CAD build for the part. Positions are in the model's coordinates, mm. A direction names the side the tool comes from. Give positions to 0.01 mm unless a question says otherwise; leave off trailing zeros. Write each loop counter-clockwise with the first axis right and the second up, starting at its lowest first coordinate (ties: lowest second). Pieces come first, ordered by that corner, then holes. Notation, with made-up numbers: (44.5, 68) - (78.5, 68) arc R17 ccw to (78.5, 99) - close; hole circle Ø1 at (1.5, -34.5). An arc over 180 degrees is marked (long way). Put each result on its own line as item: value. Start each with the question number.
1. Cut at C-C on y = 10.5. List the corners of the cut face in (x, z), and give its area (3 significant figures).
2. Cut at A-A on x = -8. List the corners of the cut face in (y, z).
3. Cut at B-B on z = -89.5. List the corners of the cut face in (x, y).
4. Wall check: line 1 (Z direction, x = 11, y = 9.25); line 2 (Z direction, x = 15, y = 2.5); line 3 (X direction, y = 0.25, z = -55.5). Give the ranges that are in metal, low to high.
5. Drop flat-ended pins along their axis: pin 1 (3 mm diameter, centred on y = 4.5, z = -20.5, fed in from -X); pin 2 (1 mm diameter, centred on y = -9.5, z = -2, fed in from -X); pin 3 (0.6 mm diameter, centred on x = 3, z = 111.5, fed in from -Y). Give the stop position or say it passes through.
6. Tool access for faces 1 (the flat face through (0, 9, 110.5)), 2 (the cylindrical face through (17, 0, 111)), 3 (the cylindrical face through (-17, 0, 111)): list every direction of +Z, -Z, +X, -X, +Y, -Y with a clear straight run to the whole face (end or side of a thin tool).
from build123d import *

# Parameters (mm, degrees)
BOSS_EXTRU_1_DEPTH = 110.5
BOSS_EXTRU_2_DEPTH = 2
ESQUISSE3_R        = 1.7
BOSS_EXTRU_3_DEPTH = 15


with BuildPart() as part:
    # Esquisse1 → Boss.-Extru.1 (new, symmetric)
    with BuildSketch(Plane.XY):
        with BuildLine():
            Line((-11.5, 12.5), (11.5, 12.5))
            ThreePointArc((11.5, 12.5), (24, 0), (11.5, -12.5))
            Line((11.5, -12.5), (-11.5, -12.5))
            ThreePointArc((-11.5, -12.5), (-24, 0), (-11.5, 12.5))
        make_face()
    extrude(amount=BOSS_EXTRU_1_DEPTH, both=True)

    # Esquisse2 → Boss.-Extru.2 (add)
    with BuildSketch(Plane.XY.offset(110.5)):
        with BuildLine():
            Line((-11, 6), (11, 6))
            ThreePointArc((11, 6), (17, 0), (11, -6))
            Line((11, -6), (-11, -6))
            ThreePointArc((-11, -6), (-17, 0), (-11, 6))
        make_face()
    extrude(amount=BOSS_EXTRU_2_DEPTH)

    # Esquisse3 → Boss.-Extru.3 (add)
    with BuildSketch(Plane.XY.offset(112.5)):
        with Locations((2.5, 0)):
            Circle(ESQUISSE3_R)
        with Locations(Location((-2.5, 0, 0), (0, 0, 180))):
            Circle(ESQUISSE3_R)
    extrude(amount=BOSS_EXTRU_3_DEPTH)


solid = part.part
Report:
1. outline: (-18.28, -110.5) - (18.28, -110.5) - (18.28, 110.5) - (-18.28, 110.5) - close
1. area: 8,080 mm²
2. outline: (-12.5, -110.5) - (12.5, -110.5) - (12.5, 110.5) - (6, 110.5) - (6, 112.5) - (-6, 112.5) - (-6, 110.5) - (-12.5, 110.5) - close
3. outline: (-11.5, -12.5) - (11.5, -12.5) arc R12.5 ccw to (11.5, 12.5) - (-11.5, 12.5) arc R12.5 ccw to start
4. line 1: z = -110.5 to 110.5
4. line 2: z = -110.5 to 112.5
4. line 3: x = -24 to 24
5. pin 1: stops at x = -23.63
5. pin 2: stops at x = -20.17
5. pin 3: stops at y = -6
6. face 1: +Z
6. face 2: +Z, +X
6. face 3: +Z, -X
